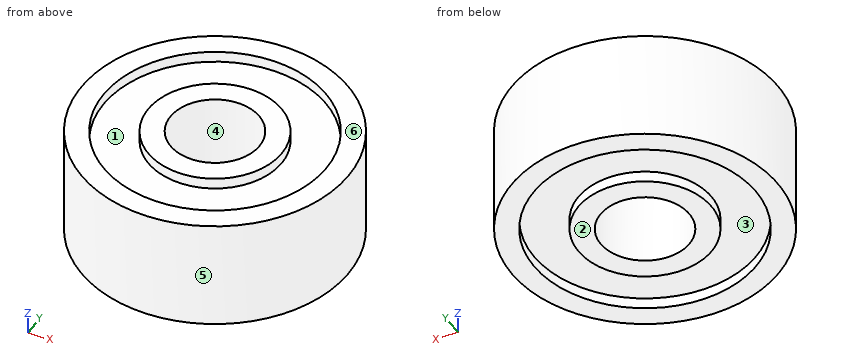
```python
from build123d import *

# Parameters (mm, degrees)
SALIENTE_EXTRUIR2_DEPTH        = 2.5
SALIENTE_EXTRUIR2_DEPTH_BACK   = 2.5
CROQUIS1_R                     = 6
CROQUIS1_R_2                   = 5
SALIENTE_EXTRUIR2_2_DEPTH      = 2.5
SALIENTE_EXTRUIR2_2_DEPTH_BACK = 2.5
CROQUIS1_R_3                   = 3
CROQUIS1_R_4                   = 2
SALIENTE_EXTRUIR3_DEPTH        = 2
SALIENTE_EXTRUIR3_DEPTH_BACK   = 2
CROQUIS1_3_R                   = 5
CROQUIS1_3_R_2                 = 3


with BuildPart() as part:
    # Croquis1 → Saliente-Extruir2 (new, two sides: drawn at the far end of the back side and taken through both)
    with BuildSketch(Plane.XY.offset(-SALIENTE_EXTRUIR2_DEPTH_BACK)):
        Circle(CROQUIS1_R)
        Circle(CROQUIS1_R_2, mode=Mode.SUBTRACT)
    extrude(amount=SALIENTE_EXTRUIR2_DEPTH + SALIENTE_EXTRUIR2_DEPTH_BACK)



with BuildPart() as body_2:
    # Croquis1 → Saliente-Extruir2 2 (new, two sides: drawn at the far end of the back side and taken through both)
    with BuildSketch(Plane.XY.offset(-SALIENTE_EXTRUIR2_2_DEPTH_BACK)):
        Circle(CROQUIS1_R_3)
        Circle(CROQUIS1_R_4, mode=Mode.SUBTRACT)
    extrude(amount=SALIENTE_EXTRUIR2_2_DEPTH + SALIENTE_EXTRUIR2_2_DEPTH_BACK)


with BuildPart() as part_1:
    add(part.part)

    add(body_2.part)  # Saliente-Extruir3 merges body 2
    # Croquis1<3> → Saliente-Extruir3 (add, two sides: drawn at the far end of the back side and taken through both)
    with BuildSketch(Plane.XY.offset(-SALIENTE_EXTRUIR3_DEPTH_BACK)):
        Circle(CROQUIS1_3_R)
        Circle(CROQUIS1_3_R_2, mode=Mode.SUBTRACT)
    extrude(amount=SALIENTE_EXTRUIR3_DEPTH + SALIENTE_EXTRUIR3_DEPTH_BACK)


solid = part_1.part
```
Build history of the part. All positions in model axes, mm. Face numbers are marked on the shaded views. A direction names the side the tool comes from. Give positions to 0.01 mm unless a question says otherwise; leave off trailing zeros. Loops run counter-clockwise (first coordinate to the right, second up) from the corner with the lowest first, then second, coordinate; pieces in that order, holes last. Notation, with made-up numbers: (81.25, 88.5) - (109.25, 88.5) arc R27 cw to (109.25, 104.5) - close; hole circle Ø2 at (28.5, -6). An arc over 180 degrees is marked (long way). Use a Markdown table: item, result.
(1) Wall check: line 1 along Y through (x, z) = (0, -2.1); line 2 along X through (y, z) = (0.25, 2.15); line 3 along Y through (x, z) = (3.75, -2.1). Give the ranges that are in metal, low to high.
Taken from the geometry:
| item | result |
|---|---|
| line 1 | -6 to -5, -3 to -2, 2 to 3, 5 to 6 |
| line 2 | -5.99 to -4.99, -2.99 to -1.98, 1.98 to 2.99, 4.99 to 5.99 |
| line 3 | -4.68 to -3.31, 3.31 to 4.68 |
(2) Which spindle directions (+Z, -Z, +X, -X, +Y, -Y) get a long thin tool onto all of the face, cutting with end or side? Do the marked faces 1, 2 and 3. Say none if no direction does.
Taken from the geometry:
| item | result |
|---|---|
| face 1 | +Z |
| face 2 | -Z, +X, -X, +Y, -Y |
| face 3 | -Z |
(3) Band-saw the part on C-C (z = -0.85). Give the cut face in (x, y).
Taken from the geometry:
| item | result |
|---|---|
| outline | circle Ø12 at (0, 0); hole circle Ø4 at (0, 0) |
(4) Band-saw the part on A-A (x = 0). Give the cut face in (y, z).
Taken from the geometry:
| item | result |
|---|---|
| outline | (-6, -2.5) - (-5, -2.5) - (-5, -2) - (-3, -2) - (-3, -2.5) - (-2, -2.5) - (-2, 2.5) - (-3, 2.5) - (-3, 2) - (-5, 2) - (-5, 2.5) - (-6, 2.5) - close; (2, -2.5) - (3, -2.5) - (3, -2) - (5, -2) - (5, -2.5) - (6, -2.5) - (6, 2.5) - (5, 2.5) - (5, 2) - (3, 2) - (3, 2.5) - (2, 2.5) - close |
(5) Band-saw the part on D-D (y = 3.25). Give the cut face in (x, z).
Taken from the geometry:
| item | result |
|---|---|
| outline | (-5.04, -2.5) - (-3.8, -2.5) - (-3.8, -2) - (3.8, -2) - (3.8, -2.5) - (5.04, -2.5) - (5.04, 2.5) - (3.8, 2.5) - (3.8, 2) - (-3.8, 2) - (-3.8, 2.5) - (-5.04, 2.5) - close |
(6) Pull direction X, two halves, no side cores. Call the marked faces 4, 5 and 6: +X half, -X half, draft (parallel to the pull), parting line (faces both ways), or undercut.
Taken from the geometry:
| item | result |
|---|---|
| face 4 | undercut |
| face 5 | parting line |
| face 6 | draft |
